from build123d import *

# Parameters (mm, degrees)
F0_W     = 60
F0_H     = 40
F1_DEPTH = 40
F2_W     = 10
F2_H     = 20
F3_DEPTH = 40
F5_DEPTH = 40


with BuildPart() as f1:
    # F0 (on Front) → F1 (new body)
    with BuildSketch(Plane.XZ):
        with Locations((-7.386366, 14.628025)):
            Rectangle(F0_W, F0_H)
    extrude(amount=F1_DEPTH)

    # F2 (on face) → F3 (cut)
    with BuildSketch(Plane(origin=(-37.386366, 0, 0), x_dir=(0, -1, 0), z_dir=(-1, 0, 0))):
        with Locations((35, 4.628025)):
            Rectangle(F2_W, F2_H)
    extrude(amount=-F3_DEPTH, mode=Mode.SUBTRACT)

    # F4 (on face) → F5 (cut)
    with BuildSketch(Plane(origin=(-37.386366, 0, 0), x_dir=(0, -1, 0), z_dir=(-1, 0, 0))):
        Polygon((40, 34.628025), (0, 34.628025), (20, 24.628025), align=None)
    extrude(amount=-F5_DEPTH, mode=Mode.SUBTRACT)


solid = f1.part
The listing builds one solid part. Answer for the finished solid, in the listing's coordinates (mm). A direction names the side the tool comes from. Coordinates: 2 decimals unless noted, no trailing zeros. Write each loop counter-clockwise with the first axis right and the second up, starting at its lowest first coordinate (ties: lowest second). Pieces come first, ordered by that corner, then holes. Notation, with made-up numbers: (-2, -1.75) - (43, -1.75) arc R18 cw to (43, 6.25) - close; hole circle Ø10 at (73, 21). An arc over 180 degrees is marked (long way). Return JSON: item names as keys, results as strings.
1. The part is cut by section C-C on y = -14.5. Determine the outline of the cut face in (x, z), then the cut area to 3 significant figures.
Final values:
{"outline": "(-37.39, -5.37) - (22.61, -5.37) - (22.61, 34.63) - (2.61, 34.63) - (2.61, 27.38) - (-37.39, 27.38) - close", "area": "2,110 mm^2"}
2. Consider line 1 along Y through (x, z) = (-9, 14.5); line 2 along X through (y, z) = (-35.5, 1); line 3 along Z through (x, y) = (-9, -25.5). Determine where each line is inside the solid, lowest interval first.
Final values:
{"line 1": "-30 to 0", "line 2": "2.61 to 22.61", "line 3": "-5.37 to 27.38"}
3. Which of the six approach directions +Z, -Z, +X, -X, +Y, -Y give full straight-line access (tool end or side, diameter ignored) to faces 1 (the face through (2.614, -20, 31)), 2 (the face through (-18, -35, 14.628)), 3 (the face through (22.614, -20, 14))?
Final values:
{"face 1": "+Z, -X", "face 2": "-Z, -X, -Y", "face 3": "+Z, -Z, +X, +Y, -Y"}
4. For a pull along Y with two mould halves and no side action, classify faces 4 (the face through (-8, 0, 15)), 5 (the face through (-17.67, -29.86, 29.56)), 6 (the face through (-1, -40, 19)), 7 (the face through (-17.67, -9.86, 29.7)) as +Y half, -Y half, draft (parallel to the pull), parting line (faces both ways), or undercut.
Final values:
{"face 4": "+Y half", "face 5": "undercut", "face 6": "-Y half", "face 7": "undercut"}
5. The part is cut by section B-B on z = -1.5. Determine the outline of the cut face in (x, y).
Final values:
{"outline": "(-37.39, -30) - (2.61, -30) - (2.61, -40) - (22.61, -40) - (22.61, 0) - (-37.39, 0) - close"}
6. Each of these flat-tipped pins is pushed along its axis until it touches: pin 1 Ø16 at (x, z) = (-11, 1) entering from -Y; pin 2 Ø8 at (y, z) = (-34.5, 5) entering from -X; pin 3 Ø2 at (x, y) = (-15, -23.5) entering from +Z. Where does it stop, or does it pass through?
Final values:
{"pin 1": "y = -30", "pin 2": "x = 2.61", "pin 3": "z = 26.88"}
7. The part is cut by section A-A on x = -28.5. Determine the outline of the cut face in (y, z), then the cut area to 3 significant figures.
Final values:
{"outline": "(-40, 14.63) - (-30, 14.63) - (-30, -5.37) - (0, -5.37) - (0, 34.63) - (-20, 24.63) - (-40, 34.63) - close", "area": "1,200 mm^2"}
